Input: part model. Units: mm. Frame: model coordinates. Give positions to 0.01 mm unless a question says otherwise; leave off trailing zeros. Order: outer loops, then holes, each group sorted by start corner. A loop starts at its lowest first (then second) coordinate and runs counter-clockwise, first axis right, second up. Notation, with made-up numbers: M 21,11 L 77,11 A20 ccw 77,27 Z; hole C 77.5,81.25 d6. An arc over 180 degrees is marked long. Use a Markdown table: item, result.
Autodesk Inventor part; units mm, degrees
ref_plane "YZ Plane" through (0, 0, 0) normal (1, 0, 0) x (0, 1, 0)
ref_plane "XZ Plane" through (0, 0, 0) normal (0, 1, 0) x (-1, 0, 0)
ref_plane "XY Plane" through (0, 0, 0) normal (0, 0, 1) x (1, 0, 0)
ref_plane "Work Plane1" through (0, 0, 0) normal (0, 0, 1) x (1, 0, 0)
sketch "Sketch1" plane through (0, 0, 0) normal (0, 0, 1) x (1, 0, 0)
  circle A0 centre (15.5, -15.5) radius 1.7
  circle A1 centre (15.5, 15.5) radius 1.7
  circle A2 centre (-15.5, 15.5) radius 1.7
  circle A3 centre (-15.5, -15.5) radius 1.7
  circle A4 centre (0, 0) radius 11
  line L0 (17.5, 21) -> (21, 17.5)
  line L1 (17.5, 21) -> (-17.5, 21)
  line L2 (-21, 17.5) -> (-17.5, 21)
  line L3 (-21, 17.5) -> (-21, -17.5)
  line L4 (-17.5, -21) -> (-21, -17.5)
  line L5 (-17.5, -21) -> (17.5, -21)
  line L6 (21, -17.5) -> (17.5, -21)
  line L7 (21, -17.5) -> (21, 17.5)
  line L8 (-31, 21) -> (239, 21)
  line L9 (239, 21) -> (239, -66)
  line L10 (239, -66) -> (-31, -66)
  line L11 (-31, -66) -> (-31, 21)
  circle A5 centre (207, 0) radius 22 construction
  line L12 (0, 0) -> (239, 0) construction
  circle A6 centre (0, 0) radius 11.5
  line L13 (104, 21) -> (104, -66) construction
  line L14 (-15.5, 15.5) -> (-31, 15.5) construction
  line L15 (207, 0) -> (207, -66) construction
  line L16 (0, 0) -> (0, -66) construction
  line L17 (219.5, -49) -> (194.5, -49)
  line L18 (194.5, -49) -> (194.5, -61)
  line L19 (194.5, -61) -> (219.5, -61)
  line L20 (219.5, -61) -> (219.5, -49)
  line L21 (219.5, -49) -> (194.5, -61) construction
  line L22 (194.5, -49) -> (219.5, -61) construction
  line L23 (219.5, -55) -> (194.5, -55) construction
  line L24 (-13.5, -61) -> (13.5, -61)
  line L25 (13.5, -61) -> (13.5, -49)
  line L26 (13.5, -49) -> (-13.5, -49)
  line L27 (-13.5, -49) -> (-13.5, -61)
  line L28 (-13.5, -61) -> (13.5, -49) construction
  line L29 (13.5, -61) -> (-13.5, -49) construction
  line L30 (170, 23) -> (166.5, 26.5)
  line L31 (170, 23) -> (170, -12)
  line L32 (166.5, -15.5) -> (170, -12)
  line L33 (166.5, -15.5) -> (131.5, -15.5)
  line L34 (128, -12) -> (131.5, -15.5)
  line L35 (128, -12) -> (128, 23)
  line L36 (131.5, 26.5) -> (128, 23)
  line L37 (131.5, 26.5) -> (166.5, 26.5)
  line L38 (127.5, 23.2071) -> (127.5, -12.2071)
  line L39 (127.5, -12.2071) -> (131.2929, -16)
  line L40 (131.2929, -16) -> (166.7071, -16)
  line L41 (166.7071, -16) -> (170.5, -12.2071)
  line L42 (170.5, -12.2071) -> (170.5, 23.2071)
  line L43 (170.5, 23.2071) -> (166.7071, 27)
  line L44 (166.7071, 27) -> (131.2929, 27)
  line L45 (131.2929, 27) -> (127.5, 23.2071)
  point P0 (-26, 15.5)
  point P1 (-26, -15.5)
  point P2 (234, 15.5)
  point P3 (234, -15.5)
  point P4 (207, -55)
  point P5 (226.5, -55)
  point P6 (187.5, -55)
  point P7 (0, -55)
  point P8 (20.5, -55)
  point P9 (-18.5, -55)
  point P10 (26, 15.5)
  point P11 (26, -15.5)
  point P12 (182, 15.5)
  point P13 (182, -15.5)
  point P14 (170.5, 21)
  point P15 (127.5, 21)
  dimension "d0" = 45
  dimension "d1" = 270
  dimension "d2" = 44
  dimension "d3" = 0.5
  dimension "d21" = 10
  dimension "d22" = 32
  dimension "d23" = 5
  dimension "d31" = 25
  dimension "d32" = 12
  dimension "d33" = 5
  dimension "d34" = 7
  dimension "d42" = 0.5
extrude "Extrusion1" add sketch "Sketch1" along normal blind 4 contours A0 | A1 | A2 | A3 | L8 L38 L39 L40 L41 L42 L9 L10 L11 L2 L3 L4 L5 L6 L7 L0 | L0 L7 L6 L5 L4 L3 L2 L1
hole "Hole1" at (207, 0, 0) direction (0, 0, 1) diameter 5.5 end through all
sketch "Sketch2" plane through (0, 0, 4) normal (0, 0, 1) x (1, 0, 0)
  circle A0 centre (15.5, -15.5) radius 1.7
  circle A1 centre (15.5, 15.5) radius 1.7
  circle A2 centre (-15.5, 15.5) radius 1.7
  circle A3 centre (-15.5, -15.5) radius 1.7
  circle A4 centre (0, 0) radius 11
  line L0 (17.5, 21) -> (21, 17.5)
  line L1 (17.5, 21) -> (-17.5, 21)
  line L2 (-21, 17.5) -> (-17.5, 21)
  line L3 (-21, 17.5) -> (-21, -17.5)
  line L4 (-17.5, -21) -> (-21, -17.5)
  line L5 (-17.5, -21) -> (17.5, -21)
  line L6 (21, -17.5) -> (17.5, -21)
  line L7 (21, -17.5) -> (21, 17.5)
  point P0 (-18.5, -55)
  point P1 (20.5, -55)
  point P2 (187.5, -55)
  point P3 (226.5, -55)
hole "Hole2" at (-15.5, -15.5, 4) at (-15.5, 15.5, 4) at (15.5, 15.5, 4) at (15.5, -15.5, 4) direction (0, 0, -1) diameter 3.4 end through all countersink diameter 6.6 countersink angle 90
fillet "Fillet1" radius 5 4 edges at (-31, 21, 2) (-31, -66, 2) (239, 21, 2) (239, -66, 2)
hole "Hole3" at (-26, -15.5, 0) at (-26, 15.5, 0) at (234, 15.5, 0) at (234, -15.5, 0) at (26, 15.5, 0) at (26, -15.5, 0) at (182, -15.5, 0) at (182, 15.5, 0) direction (0, 0, 1) diameter 3.4 end through all countersink diameter 6.6 countersink angle 90
hole "Hole4" at (-18.5, -55, 4) at (20.5, -55, 4) at (187.5, -55, 4) at (226.5, -55, 4) direction (0, 0, -1) diameter 3.4 end through all countersink diameter 6.6 countersink angle 90
properties part number "plate_1"
1) First-contact query: pin 1 Ø5.5 at (x, y) = (26, 15.5) entering from +Z; pin 2 Ø5.5 at (x, y) = (15.5, -15.5) entering from +Z; pin 3 Ø2 at (x, y) = (26, -15.5) entering from -Z; pin 4 Ø4 at (x, y) = (-26, -15.5) entering from -Z. Flat tips, straight axial feed; report the tip coordinate or a pass-through.
Response values:
| item | result |
|---|---|
| pin 1 | stops at z = 4 |
| pin 2 | stops at z = 3.45 |
| pin 3 | passes through |
| pin 4 | stops at z = 1.3 |
2) Mould query, pull axis Y, two halves, no side actions, for faces 1 (the face through (238, 19, 2)), 2 (the face through (209.685, -0.596, 2.028)), 3 (the face through (102, -22, 4)). Classes: released by +Y, released by -Y, zero draft, split by the parting line, or undercut.
Response values:
| item | result |
|---|---|
| face 1 | released by +Y |
| face 2 | undercut |
| face 3 | zero draft |
3) Material intervals for line 1 (X direction, y = -57, z = 1.65); line 2 (Y direction, x = 182, z = 2.5); line 3 (X direction, y = -0.5, z = 1.75), sorted ascending. Write a range as from..to.
Response values:
| item | result |
|---|---|
| line 1 | x = -31..-13.5, 13.5..194.5, 219.5..239 |
| line 2 | y = -66..-17.2, -13.8..13.8, 17.2..21 |
| line 3 | x = -31..-11.49, 11.49..127.5, 170.5..204.3, 209.7..239 |
4) Cut plane B-B on x = 207. Return loops of the section in (y, z).
Response values:
| item | result |
|---|---|
| outline | M -66,0 L -61,0 L -61,4 L -66,4 Z; M -49,0 L -2.75,0 L -2.75,4 L -49,4 Z; M 2.75,0 L 21,0 L 21,4 L 2.75,4 Z |
5) Cut plane A-A on y = 0. Return loops of the section in (x, z), and give its area (3 significant figures).
Response values:
| item | result |
|---|---|
| outline | M -31,0 L -11.5,0 L -11.5,4 L -31,4 Z; M 11.5,0 L 127.5,0 L 127.5,4 L 11.5,4 Z; M 170.5,0 L 204.25,0 L 204.25,4 L 170.5,4 Z; M 209.75,0 L 239,0 L 239,4 L 209.75,4 Z |
| area | 794 mm² |
6) Cut plane C-C on z = 1. State how many separate pieces and enclosed holes the cut face has, and give its area (3 significant figures).
Response values:
| item | result |
|---|---|
| separate pieces | 1 |
| enclosed holes | 20 |
| area | 20,600 mm² |
